```python
from build123d import *

# Parameters (mm, degrees)
CROQUIS1_R              = 2.5
SALIENTE_EXTRUIR1_DEPTH = 2
CROQUIS2_R              = 1.5
SALIENTE_EXTRUIR2_DEPTH = 15
CHAFL_N1_SIZE           = 0.25
REDONDEO1_R             = 0.5
CORTAR_EXTRUIR1_DEPTH   = 1
CHAFL_N2_SIZE           = 0.25
CHAFL_N2_SIZE2          = 0.933012702


with BuildPart() as part:
    # Croquis1 → Saliente-Extruir1 (new body)
    with BuildSketch(Plane(origin=(0, 0, 0), x_dir=(1, 0, 0), z_dir=(0, 1, 0))):
        Circle(CROQUIS1_R)
    extrude(amount=SALIENTE_EXTRUIR1_DEPTH)

    # Croquis2 → Saliente-Extruir2 (add)
    with BuildSketch(Plane.XZ):
        Circle(CROQUIS2_R)
    extrude(amount=SALIENTE_EXTRUIR2_DEPTH)

    # Chaflán1
    chafl_n1_edges = [part.edges().sort_by_distance(p)[0] for p in [
        (-2.5, 0, 0),
        (-1.5, -15, 0),
    ]]
    chamfer(chafl_n1_edges, length=CHAFL_N1_SIZE)

    # Redondeo1
    redondeo1_edges = [part.edges().sort_by_distance(p)[0] for p in [
        (-2.5, 2, 0),
    ]]
    fillet(redondeo1_edges, radius=REDONDEO1_R)

    # Croquis3 → Cortar-Extruir1 (cut)
    with BuildSketch(Plane(origin=(0, 2, 0), x_dir=(1, 0, 0), z_dir=(0, 1, 0))):
        Polygon((0.25, 0.25), (1.45, 0.25), (1.45, -0.25), (0.25, -0.25), (0.25, -1.45), (-0.25, -1.45), (-0.25, -0.25), (-1.45, -0.25), (-1.45, 0.25), (-0.25, 0.25), (-0.25, 1.45), (0.25, 1.45), align=None)
    extrude(amount=-CORTAR_EXTRUIR1_DEPTH, mode=Mode.SUBTRACT)

    # Chaflán2
    chafl_n2_edges = [part.edges().sort_by_distance(p)[0] for p in [
        (-0.25, 2, -0.85),
        (-0.85, 2, -0.25),
        (-0.85, 2, 0.25),
        (-0.25, 2, 0.85),
        (0.25, 2, 0.85),
        (0.85, 2, 0.25),
        (0.85, 2, -0.25),
        (0.25, 2, -0.85),
    ]]
    chafl_n2_side = [part.faces().sort_by_distance(p)[0] for p in [
        (-1.943431458, 2, 0),
    ]]
    chamfer(chafl_n2_edges, length=CHAFL_N2_SIZE, length2=CHAFL_N2_SIZE2, reference=chafl_n2_side[0])


solid = part.part
```
Could you check a few things on this model? Use its own coordinates, in mm. A direction names the side the tool comes from. Coordinates: 2 decimals unless noted, no trailing zeros. Order: outer loops, then holes, each group sorted by start corner. A loop starts at its lowest first (then second) coordinate and runs counter-clockwise, first axis right, second up. Notation, with made-up numbers: M -6,75.25 L 45,75.25 A32 ccw 45,109.25 Z; hole C -14,61 d3. An arc over 180 degrees is marked long. Use one line per item in the form item = value. Start each with the question number.
1. For pin 1 (2 mm diameter, centred on x = -1, y = -2, fed in from +Z); pin 2 (2 mm diameter, centred on x = 0.5, y = -6.5, fed in from -Z), each with a flat end and sliding along its axis, tell me the tip position at first contact or that it passes through.
2. On a 3-axis mill with a long thin cutter (end or side, diameter ignored), from which of +Z, -Z, +X, -X, +Y, -Y can I reach the whole of each face in a straight line? I mean faces 1 (the flat face through (-0.373, 1.527, 0.858)), 2 (the flat face through (0, -15, 0)). Say none if no direction works.
3. Suppose I cut it at B-B on z = 0. Write out the boundary of the cut face in (x, y).
4. Suppose I cut it at A-A on x = 0. Write out the boundary of the cut face in (y, z).
5. Please list where these lines run through material, in increasing order: line 1 (X direction, y = -9, z = -0.05); line 2 (Y direction, x = -0.8, z = 0.05).
6. We'd pull the mould along Z, two halves only. Please class faces 3 (the flat face through (-0.842, 1.527, 0.373)), 4 (the cylindrical face through (-1.5, -7.27, 0.07)), 5 (the flat face through (1, 2, 1)), 6 (the flat face through (-0.373, 1.527, -0.842)): +Z half, -Z half, draft (parallel to the pull), parting line (faces both ways), or undercut.
7. Suppose I cut it at C-C on y = -6.5. Write out the boundary of the cut face in (x, z), then the cut area to 3 significant figures.
Geometry says:
q1.pin_1 = 1.5
q1.pin_2 = -1.5
q2.face_1 = +Y
q2.face_2 = +Z, -Z, +X, -X, -Y
q3.outline = M -2.5,0.25 L -2.25,0 L -1.5,0 L -1.5,-14.75 L -1.25,-15 L 1.25,-15 L 1.5,-14.75 L 1.5,0 L 2.25,0 L 2.5,0.25 L 2.5,1.5 A0.5 ccw 2,2 L 1.45,2 L 1.45,1 L -1.45,1 L -1.45,2 L -2,2 A0.5 ccw -2.5,1.5 Z
q4.outline = M -15,-1.25 L -14.75,-1.5 L 0,-1.5 L 0,-2.25 L 0.25,-2.5 L 1.5,-2.5 A0.5 ccw 2,-2 L 2,-1.45 L 1,-1.45 L 1,1.45 L 2,1.45 L 2,2 A0.5 ccw 1.5,2.5 L 0.25,2.5 L 0,2.25 L 0,1.5 L -14.75,1.5 L -15,1.25 Z
q5.line_1 = -1.5 to 1.5
q5.line_2 = -15 to 1
q6.face_3 = undercut
q6.face_4 = parting line
q6.face_5 = draft
q6.face_6 = undercut
q7.outline = C 0,0 d3
q7.area = 7.07 mm^2
